Could you check a few things on this model? Use its own coordinates, in mm. A direction names the side the tool comes from. Coordinates: 2 decimals unless noted, no trailing zeros. Loops run counter-clockwise (first coordinate to the right, second up) from the corner with the lowest first, then second, coordinate; pieces in that order, holes last. Notation, with made-up numbers: M 42.5,44 L 57.5,44 A3 cw 57.5,49 Z; hole C 75,10.25 d2. An arc over 180 degrees is marked long. Return JSON: item names as keys, results as strings. Group by question number.
from build123d import *

# Parameters (mm, degrees)
BOSS_EXTRUDE1_DEPTH = 15
CHAMFER1_SIZE       = 2
FILLET1_R           = 2
FILLET3_R           = 5
FILLET4_R           = 0.5


with BuildPart() as part:
    # Sketch2 → Boss-Extrude1 (new body)
    with BuildSketch(Plane(origin=(0, 0, 0), x_dir=(1, 0, 0), z_dir=(0, 1, 0))):
        Polygon((-14.166102689, -0.628958771), (-9.166102689, -0.628958771), (-11.166102689, 1.371041229), (-11.166102689, 7.371041229), (-9.166102689, 9.371041229), (-9.166102689, 14.371041229), (-3.066102689, 14.371041229), (-3.066102689, 9.371041229), (-1.066102689, 7.371041229), (-1.066102689, 1.371041229), (-3.066102689, -0.628958771), (1.933897311, -0.628958771), (1.933897311, 10.071041229), (-0.066102689, 11.631429668), (-0.066102689, 18.371041229), (-12.166102689, 18.371041229), (-12.166102689, 11.631429668), (-14.166102689, 10.071041229), align=None)
    extrude(amount=BOSS_EXTRUDE1_DEPTH)

    # Chamfer1
    chamfer1_edges = [part.edges().sort_by_distance(p)[0] for p in [
        (-14.166102689, 7.5, 0.628958771),
        (1.933897311, 7.5, 0.628958771),
    ]]
    chamfer(chamfer1_edges, length=CHAMFER1_SIZE)

    # Fillet1
    fillet1_edges = [part.edges().sort_by_distance(p)[0] for p in [
        (-3.066102689, 7.5, -14.371041229),
        (-9.166102689, 7.5, -14.371041229),
    ]]
    fillet(fillet1_edges, radius=FILLET1_R)

    # Fillet3
    fillet3_edges = [part.edges().sort_by_distance(p)[0] for p in [
        (-12.166102689, 7.5, -18.371041229),
        (-0.066102689, 7.5, -18.371041229),
    ]]
    fillet(fillet3_edges, radius=FILLET3_R)

    # Fillet4
    fillet4_edges = [part.edges().sort_by_distance(p)[0] for p in [
        (-9.166102689, 7.5, 0.628958771),
        (-3.066102689, 7.5, 0.628958771),
    ]]
    fillet(fillet4_edges, radius=FILLET4_R)


solid = part.part
(1) If I drill on L1, parallel to X at y = 13, z = -6.5; L2, parallel to X at y = 10.75, z = -10; L3, parallel to Z at x = -6, y = 1.75, over which ranges is the centre line in solid material (lowest first)? Write a range as [from, to].
(2) Will these pins go through, and if not, where does the flat tip stop? P1, Ø1.4, axis at y = 5.5, z = -13, coming from the +X side; P2, Ø4, axis at x = -3.5, z = -3.5, coming from the -Y side; P3, Ø1.7, axis at x = -6, y = 7, coming from the +Z side; P4, Ø1, axis at y = 9, z = -13.5, coming from the -X side.
(3) Imagine slicing it at B-B, the plane y = 6. Write out the boundary of the cut face in (x, z).
(4) Imagine slicing it at C-C, the plane z = -8.75. Write out the boundary of the cut face in (x, y).
(5) Imagine slicing it at D-D, the plane x = 1. Write out the boundary of the cut face in (y, z), then the cut area to 3 significant figures.
(6) We'd pull the mould along Z, two halves only. Please class faces 6 (the face through (-0.066, 7, -12)), 7 (the face through (0.948, 7.395, -0.385)), 8 (the face through (-1.066, 7, -4)): +Z half, -Z half, draft (parallel to the pull), parting line (faces both ways), or undercut.
(7) Imagine slicing it at A-A, the plane z = -3.5. Write out the boundary of the cut face in (x, y).
(8) For faces 1 (the face through (-9.914, 7.605, 0.328)), 2 (the face through (1.934, 7, -6)), 3 (the face through (-13.18, 7.395, -0.385)), 4 (the face through (-3.066, 7, -11)), 5 (the face through (-12.166, 7, -13)), which set-ups out of +Z, -Z, +X, -X, +Y, -Y let a thin tool reach every point of the face, with its end or its side?
Checks:
{
 "1": {"L1": "[-14.17, -11.17], [-1.07, 1.93]", "L2": "[-14.17, -9.17], [-3.07, 1.93]", "L3": "[-18.37, -14.37]"},
 "2": {"P1": "x = -0.07", "P2": "through", "P3": "z = -14.37", "P4": "x = -12.17"},
 "3": {"outline": "M -14.17,-10.07 L -12.17,-11.63 L -12.17,-13.37 A5 ccw -7.17,-18.37 L -5.07,-18.37 A5 ccw -0.07,-13.37 L -0.07,-11.63 L 1.93,-10.07 L 1.93,-1.37 L -0.07,0.63 L -1.86,0.63 A0.5 ccw -2.21,-0.22 L -1.07,-1.37 L -1.07,-7.37 L -3.07,-9.37 L -3.07,-12.37 A2 cw -5.07,-14.37 L -7.17,-14.37 A2 cw -9.17,-12.37 L -9.17,-9.37 L -11.17,-7.37 L -11.17,-1.37 L -10.02,-0.22 A0.5 ccw -10.37,0.63 L -12.17,0.63 L -14.17,-1.37 Z"},
 "4": {"outline": "M -14.17,0 L -9.79,0 L -9.79,15 L -14.17,15 Z; M -2.45,0 L 1.93,0 L 1.93,15 L -2.45,15 Z"},
 "5": {"outline": "M 0,-10.8 L 15,-10.8 L 15,-0.44 L 0,-0.44 Z", "area": "155 mm²"},
 "6": {"face 6": "draft", "face 7": "+Z half", "face 8": "undercut"},
 "7": {"outline": "M -14.17,0 L -11.17,0 L -11.17,15 L -14.17,15 Z; M -1.07,0 L 1.93,0 L 1.93,15 L -1.07,15 Z"},
 "8": {"face 1": "+Y, -Y", "face 2": "+Z, -Z, +X, +Y, -Y", "face 3": "+Z, -X, +Y, -Y", "face 4": "+Z, +Y, -Y", "face 5": "-Z, -X, +Y, -Y"}
}
